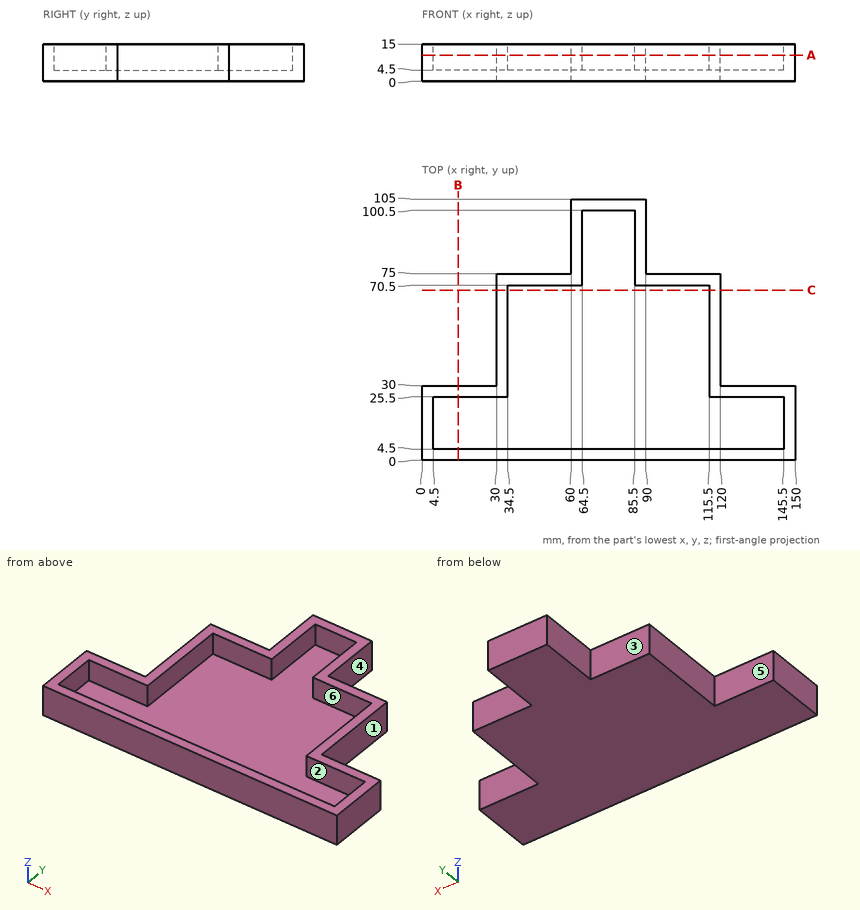
Input: dimensioned drawing with shaded views. Units: mm. Origin: part minimum x, y, z. A direction names the side the tool comes from. Round coordinates to 2 decimals unless told otherwise and drop trailing zeros. Order: outer loops, then holes, each group sorted by start corner. A loop starts at its lowest first (then second) coordinate and runs counter-clockwise, first axis right, second up.
Q1. Section A-A, the plane z = 10.5. Output: boundary loops of the cut face in (x, y).
Result sheet:
outline: (0, 0) - (150, 0) - (150, 30) - (120, 30) - (120, 75) - (90, 75) - (90, 105) - (60, 105) - (60, 75) - (30, 75) - (30, 30) - (0, 30) - close; hole (4.5, 4.5) - (145.5, 4.5) - (145.5, 25.5) - (115.5, 25.5) - (115.5, 70.5) - (85.5, 70.5) - (85.5, 100.5) - (64.5, 100.5) - (64.5, 70.5) - (34.5, 70.5) - (34.5, 25.5) - (4.5, 25.5) - close
Q2. Pin query (flat end, axial travel): pin 1 (8.5 mm diameter, centred on y = 87, z = 11, fed in from +X); pin 2 (8.5 mm diameter, centred on y = 49.5, z = 8.5, fed in from -X); pin 3 (5 mm diameter, centred on y = 47, z = 11, fed in from +X). Return the tip coordinate at first contact, or that it passes through.
Result sheet:
pin 1: stops at x = 90
pin 2: stops at x = 30
pin 3: stops at x = 120
Q3. Access query for the marked faces 4, 5 and 6. Directions: +Z, -Z, +X, -X, +Y, -Y. A direction counts if a zero-diameter tool reaches every point of the face in a straight line with its end or side. Return the directions, or none.
Result sheet:
face 4: +Z, -Z, +X, +Y
face 5: +Z, -Z, -X, +Y
face 6: +Z
Q4. Mould query, pull axis X, two halves, no side actions, for the marked faces 1, 2 and 3. Classes: released by +X, released by -X, zero draft, split by the parting line, or undercut.
Result sheet:
face 1: released by +X
face 2: undercut
face 3: zero draft
Q5. Material intervals for probe 1 along X at (y, z) = (81, 6); probe 2 along X at (y, z) = (57.5, 6.25); probe 3 along Y at (x, z) = (49.5, 5.25), sorted ascending.
Result sheet:
probe 1: x = 60 to 64.5, 85.5 to 90
probe 2: x = 30 to 34.5, 115.5 to 120
probe 3: y = 0 to 4.5, 70.5 to 75
Q6. Section B-B, the plane x = 14.5. Output: boundary loops of the cut face in (y, z), and give its area (4 significant figures).
Result sheet:
outline: (0, 0) - (30, 0) - (30, 15) - (25.5, 15) - (25.5, 4.5) - (4.5, 4.5) - (4.5, 15) - (0, 15) - close
area: 229.5 mm2
Q7. Section C-C, the plane y = 68.5. Output: boundary loops of the cut face in (x, z), and give its area (4 significant figures).
Result sheet:
outline: (30, 0) - (120, 0) - (120, 15) - (115.5, 15) - (115.5, 4.5) - (34.5, 4.5) - (34.5, 15) - (30, 15) - close
area: 499.5 mm2
